Verification items for this drawing (mm, ordinates from the low corner). A direction names the side the tool comes from. Give positions to 0.01 mm unless a question says otherwise; leave off trailing zeros. Loops run counter-clockwise (first coordinate to the right, second up) from the corner with the lowest first, then second, coordinate; pieces in that order, holes last. Notation, with made-up numbers: M 50,25 L 96,25 A23 cw 96,61 Z; hole C 80,58 d6. An arc over 180 degrees is marked long. Answer in a Markdown table with one row per item.
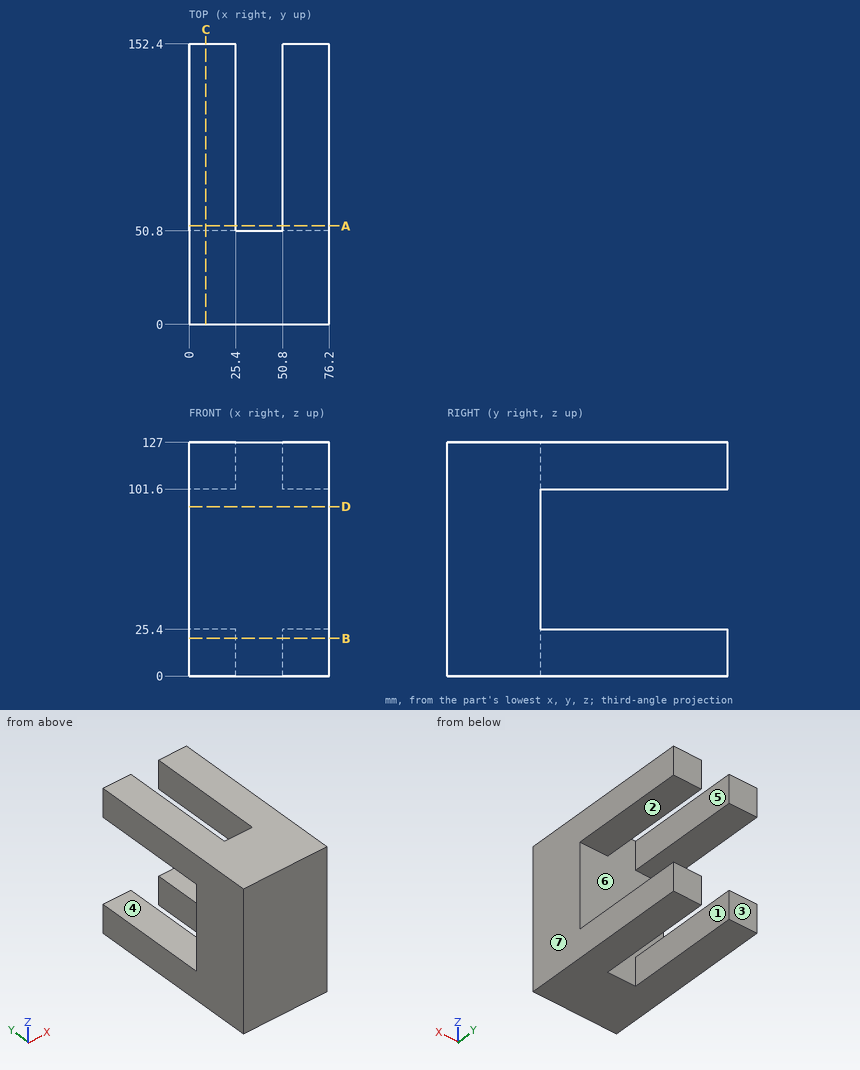
Item 1: Tool access check on the marked faces 1, 2 and 3. Record the directions out of +Z, -Z, +X, -X, +Y, -Y that give a thin tool (end or side, any length) a straight path to the whole face; none if there is none.
Reported:
| item | result |
|---|---|
| face 1 | +Z, -Z, +Y |
| face 2 | +X, -X, +Y |
| face 3 | +Z, -Z, +X, -X, +Y |
Item 2: Sectioned sample at A-A (y = 53.5). Record the cut outline in (x, z), and give its area (3 significant figures).
Reported:
| item | result |
|---|---|
| outline | M 0,0 L 25.4,0 L 25.4,25.4 L 0,25.4 Z; M 0,101.6 L 25.4,101.6 L 25.4,127 L 0,127 Z; M 50.8,0 L 76.2,0 L 76.2,25.4 L 50.8,25.4 Z; M 50.8,101.6 L 76.2,101.6 L 76.2,127 L 50.8,127 Z |
| area | 2,580 mm^2 |
Item 3: Sectioned sample at B-B (z = 20.5). Record the cut outline in (x, y), and give its area (3 significant figures).
Reported:
| item | result |
|---|---|
| outline | M 0,0 L 76.2,0 L 76.2,152.4 L 50.8,152.4 L 50.8,50.8 L 25.4,50.8 L 25.4,152.4 L 0,152.4 Z |
| area | 9,030 mm^2 |
Item 4: Release check for a two-part mould opening along X. For the marked faces 4, 5, 6 and 7 record: released by +X, released by -X, zero draft, split by the parting line, or undercut.
Reported:
| item | result |
|---|---|
| face 4 | zero draft |
| face 5 | undercut |
| face 6 | undercut |
| face 7 | released by +X |
Item 5: Scan lines: L1, parallel to Z at x = 62.5, y = 84.5; L2, parallel to X at y = 75.5, z = 106; L3, parallel to Y at x = 25.5, z = 98. Record each from-to range of solid material in increasing order. Write a range as [from, to].
Reported:
| item | result |
|---|---|
| L1 | z = [0, 25.4], [101.6, 127] |
| L2 | x = [0, 25.4], [50.8, 76.2] |
| L3 | y = [0, 50.8] |
Item 6: Sectioned sample at C-C (x = 9). Record the cut outline in (y, z).
Reported:
| item | result |
|---|---|
| outline | M 0,0 L 152.4,0 L 152.4,25.4 L 50.8,25.4 L 50.8,101.6 L 152.4,101.6 L 152.4,127 L 0,127 Z |
Item 7: Sectioned sample at D-D (z = 92). Record the cut outline in (x, y).
Reported:
| item | result |
|---|---|
| outline | M 0,0 L 76.2,0 L 76.2,50.8 L 0,50.8 Z |
